CAD build for the part. Positions are in the model's coordinates, mm. Face numbers are marked on the shaded views. Give positions to 0.01 mm unless a question says otherwise; leave off trailing zeros. Loops run counter-clockwise (first coordinate to the right, second up) from the corner with the lowest first, then second, coordinate; pieces in that order, holes last. Notation, with made-up numbers: M 9,56 L 43,56 A14 cw 43,73 Z; hole C 7,42 d7. An arc over 180 degrees is marked long. Answer as CSV lines item,"result".
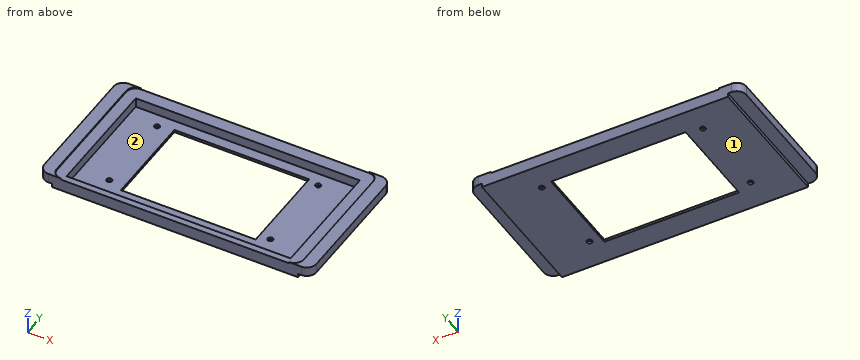
```python
from build123d import *

# Parameters (mm, degrees)
BOSS_EXTRUDE1_DEPTH       = 10.5
CUT_EXTRUDE1_DEPTH        = 1
M5X0_8_TAPPED_HOLE1_D     = 4.2
M5X0_8_TAPPED_HOLE1_DEPTH = 12.4
M5X0_8_TAPPED_HOLE1_TIP   = 1.2618073
SKETCH7_W                 = 105.52
SKETCH7_H                 = 73.399079938
CUT_EXTRUDE2_DEPTH        = 121.239344642
SKETCH9_W                 = 175.5
SKETCH9_H                 = 95
CUT_EXTRUDE3_DEPTH        = 7.5
CUT_EXTRUDE4_START        = -3
CUT_EXTRUDE4_DEPTH        = 3


with BuildPart() as part:
    # Sketch1 → Boss-Extrude1 (new body)
    with BuildSketch(Plane.XY):
        with BuildLine():
            Line((-99, 55), (99, 55))
            ThreePointArc((99, 55), (104.303300859, 52.803300859), (106.5, 47.5))
            Line((106.5, 47.5), (106.5, -47.5))
            ThreePointArc((106.5, -47.5), (104.303300859, -52.803300859), (99, -55))
            Line((99, -55), (-99, -55))
            ThreePointArc((-99, -55), (-104.303300859, -52.803300859), (-106.5, -47.5))
            Line((-106.5, -47.5), (-106.5, 47.5))
            ThreePointArc((-106.5, 47.5), (-104.303300859, 52.803300859), (-99, 55))
        make_face()
    extrude(amount=-BOSS_EXTRUDE1_DEPTH)

    # Sketch2 → Cut-Extrude1 (cut)
    with BuildSketch(Plane.XY):
        with BuildLine():
            Line((-89.25, 55), (89.25, 55))
            ThreePointArc((89.25, 55), (94.553300859, 52.803300859), (96.75, 47.5))
            Line((96.75, 47.5), (96.75, -47.5))
            ThreePointArc((96.75, -47.5), (94.553300859, -52.803300859), (89.25, -55))
            Line((89.25, -55), (-89.25, -55))
            ThreePointArc((-89.25, -55), (-94.553300859, -52.803300859), (-96.75, -47.5))
            Line((-96.75, -47.5), (-96.75, 47.5))
            ThreePointArc((-96.75, 47.5), (-94.553300859, 52.803300859), (-89.25, 55))
        make_face()
    extrude(amount=-CUT_EXTRUDE1_DEPTH, mode=Mode.SUBTRACT)

    # M5x0.8 Tapped Hole1
    with Locations(Plane.XY.offset(-1)):
        with Locations((-64.86, 34.2), (61.34, 34.2), (61.34, -31.45), (-64.86, -31.45)):
            Hole(M5X0_8_TAPPED_HOLE1_D / 2, depth=M5X0_8_TAPPED_HOLE1_DEPTH)
            with Locations((0, 0, -(M5X0_8_TAPPED_HOLE1_DEPTH + M5X0_8_TAPPED_HOLE1_TIP / 2))):  # 118° drill point
                Cone(0, M5X0_8_TAPPED_HOLE1_D / 2, M5X0_8_TAPPED_HOLE1_TIP, mode=Mode.SUBTRACT)

    # Sketch7 → Cut-Extrude2 (cut, through all)
    with BuildSketch(Plane.XY.offset(-1)):
        Rectangle(SKETCH7_W, SKETCH7_H)
    extrude(amount=-CUT_EXTRUDE2_DEPTH, mode=Mode.SUBTRACT)

    # Sketch9 → Cut-Extrude3 (cut)
    with BuildSketch(Plane.XY.offset(-1)):
        with Locations((0, -2.5)):
            Rectangle(SKETCH9_W, SKETCH9_H)
    extrude(amount=-CUT_EXTRUDE3_DEPTH, mode=Mode.SUBTRACT)

    # Sketch10 → Cut-Extrude4 (cut)
    with BuildSketch(Plane(origin=(0, 0, -10.5), x_dir=(-1, 0, 0), z_dir=(0, 0, -1)).offset(CUT_EXTRUDE4_START)):
        with BuildLine():
            Line((-96.4, 55), (-99, 55))
            ThreePointArc((-99, 55), (-104.303300859, 52.803300859), (-106.5, 47.5))
            Line((-106.5, 47.5), (-106.5, -47.5))
            ThreePointArc((-106.5, -47.5), (-104.303300859, -52.803300859), (-99, -55))
            Line((-99, -55), (-96.4, -55))
            Line((-96.4, -55), (-96.4, 55))
        make_face()
        with BuildLine():
            Line((96.4, -55), (99, -55))
            ThreePointArc((99, -55), (104.303300859, -52.803300859), (106.5, -47.5))
            Line((106.5, -47.5), (106.5, 47.5))
            ThreePointArc((106.5, 47.5), (104.303300859, 52.803300859), (99, 55))
            Line((99, 55), (96.4, 55))
            Line((96.4, 55), (96.4, -55))
        make_face()
    extrude(amount=CUT_EXTRUDE4_DEPTH, mode=Mode.SUBTRACT)


solid = part.part
```
Q1. Pin check, flat tips, straight feed: P1, Ø3.5, axis at x = -64.86, y = -31.45, coming from the -Z side; P2, Ø6.5, axis at x = -64.86, y = 34.2, coming from the +Z side; P3, Ø1.6, axis at y = -5.5, z = -9.5, coming from the -X side; P4, Ø11, axis at x = -103.5, y = -1.5, coming from the -Z side. Stop position of each tip, or through.
Solution:
P1,"passes through"
P2,"stops at z = -8.5"
P3,"stops at x = -96.4"
P4,"stops at z = -7.5"
Q2. Cut at D-D (y = 17). Write the cut outline in (x, z), and give its area (3 significant figures).
Solution:
outline,"M -106.5,-7.5 L -96.4,-7.5 L -96.4,-10.5 L -52.76,-10.5 L -52.76,-8.5 L -87.75,-8.5 L -87.75,-1 L -96.75,-1 L -96.75,0 L -106.5,0 Z; M 52.76,-10.5 L 96.4,-10.5 L 96.4,-7.5 L 106.5,-7.5 L 106.5,0 L 96.75,0 L 96.75,-1 L 87.75,-1 L 87.75,-8.5 L 52.76,-8.5 Z"
area,"455 mm²"
Q3. Cut at C-C (x = 61.34). Write the cut outline in (y, z), and give its area (3 significant figures).
Solution:
outline,"M -55,-10.5 L -33.55,-10.5 L -33.55,-8.5 L -50,-8.5 L -50,-1 L -55,-1 Z; M -29.35,-10.5 L 32.1,-10.5 L 32.1,-8.5 L -29.35,-8.5 Z; M 36.3,-10.5 L 55,-10.5 L 55,-1 L 45,-1 L 45,-8.5 L 36.3,-8.5 Z"
area,"316 mm²"
Q4. Mould opens along X. For the marked faces 1 and 2 say: released by +X, released by -X, zero draft, split by the parting line, or undercut.
Solution:
face 1,"zero draft"
face 2,"undercut"
Q5. Cut at B-B (y = -31.45). Write the cut outline in (x, z), and give its area (3 significant figures).
Solution:
outline,"M -106.5,-7.5 L -96.4,-7.5 L -96.4,-10.5 L -66.96,-10.5 L -66.96,-8.5 L -87.75,-8.5 L -87.75,-1 L -96.75,-1 L -96.75,0 L -106.5,0 Z; M -62.76,-10.5 L -52.76,-10.5 L -52.76,-8.5 L -62.76,-8.5 Z; M 52.76,-10.5 L 59.24,-10.5 L 59.24,-8.5 L 52.76,-8.5 Z; M 63.44,-10.5 L 96.4,-10.5 L 96.4,-7.5 L 106.5,-7.5 L 106.5,0 L 96.75,0 L 96.75,-1 L 87.75,-1 L 87.75,-8.5 L 63.44,-8.5 Z"
area,"438 mm²"
Q6. Cut at A-A (x = 40). Write the cut outline in (y, z), and give its area (3 significant figures).
Solution:
outline,"M -55,-10.5 L -36.7,-10.5 L -36.7,-8.5 L -50,-8.5 L -50,-1 L -55,-1 Z; M 36.7,-10.5 L 55,-10.5 L 55,-1 L 45,-1 L 45,-8.5 L 36.7,-8.5 Z"
area,"186 mm²"
Q7. Wall check: line 1 (Y direction, x = -64.86, z = -9.25); line 2 (X direction, y = -19, z = -4); line 3 (Y direction, x = 86, z = -4). Give the ranges that are in metal, low to high. Write a range as [from, to].
Solution:
line 1,"y = [-55, -33.55], [-29.35, 32.1], [36.3, 55]"
line 2,"x = [-106.5, -87.75], [87.75, 106.5]"
line 3,"y = [-55, -50], [45, 55]"
